from build123d import *

# Parameters (mm, degrees)
SKETCH1_W                 = 50.8
SKETCH1_H                 = 76.2
BOSS_EXTRUDE1_DEPTH       = 2.9972
SKETCH2_W                 = 2.9972
SKETCH2_H                 = 12.7
BOSS_EXTRUDE2_DEPTH       = 2.9972
F_8_CLEARANCE_HOLE1_D     = 4.3053
F_8_CLEARANCE_HOLE1_DEPTH = 6.351016
SKETCH6_R                 = 4.7625
CUT_EXTRUDE1_DEPTH        = 48.612962265


with BuildPart() as part:
    # Sketch1 → Boss-Extrude1 (new body)
    with BuildSketch(Plane(origin=(0, 0, 0), x_dir=(1, 0, 0), z_dir=(0, 1, 0))):
        Rectangle(SKETCH1_W, SKETCH1_H)
    extrude(amount=BOSS_EXTRUDE1_DEPTH)

    # Sketch2 → Boss-Extrude2 (add)
    with BuildSketch(Plane(origin=(0, 2.9972, 0), x_dir=(1, 0, 0), z_dir=(0, 1, 0))):
        with Locations((26.8986, 31.75)):
            Rectangle(SKETCH2_W, SKETCH2_H)
        with Locations((26.8986, -31.75)):
            Rectangle(SKETCH2_W, SKETCH2_H)
        with Locations((-26.8986, -31.75)):
            Rectangle(SKETCH2_W, SKETCH2_H)
        with Locations((-26.8986, 31.75)):
            Rectangle(SKETCH2_W, SKETCH2_H)
    extrude(amount=-BOSS_EXTRUDE2_DEPTH)

    # #8 Clearance Hole1
    with Locations(Plane(origin=(0, 2.9972, 0), x_dir=(1, 0, 0), z_dir=(0, 1, 0))):
        with Locations((12.7, -25.4), (0, -25.4), (-12.7, -25.4), (-12.7, -12.7), (0, -12.7), (12.7, -12.7), (-12.7, 0), (0, 0), (12.7, 0), (12.7, 12.7), (0, 12.7), (-12.7, 12.7), (-12.7, 25.4), (0, 25.4), (12.7, 25.4)):
            Hole(F_8_CLEARANCE_HOLE1_D / 2, depth=F_8_CLEARANCE_HOLE1_DEPTH)

    # Sketch6 → Cut-Extrude1 (cut, through all)
    with BuildSketch(Plane(origin=(0, 2.9972, 0), x_dir=(1, 0, 0), z_dir=(0, 1, 0))):
        with Locations(Location((0, 0, 0), (0, 0, 270))):
            Circle(SKETCH6_R)
    extrude(amount=-CUT_EXTRUDE1_DEPTH, mode=Mode.SUBTRACT)


solid = part.part
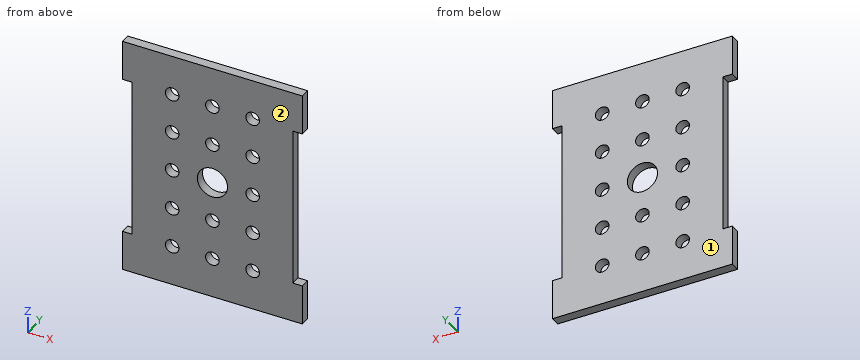
Build history of the part. All positions in model axes, mm. Face numbers are marked on the shaded views. Coordinates: 2 decimals unless noted, no trailing zeros. Write each loop counter-clockwise with the first axis right and the second up, starting at its lowest first coordinate (ties: lowest second). Pieces come first, ordered by that corner, then holes. Notation, with made-up numbers: (7.5, 43) -> (18.5, 43) arc R32 cw to (18.5, 80) -> close; hole circle Ø11 at (-27.75, 24.5). An arc over 180 degrees is marked (long way). Use CSV: the item, a comma, the result in double quotes. Start each with the question number.
Q1. Cut at A-A, the plane x = 0. List the corners of the cut face in (y, z).
Q2. Cut at C-C, the plane y = 2.45. State how many separate pieces and enclosed holes the cut face has, then the cut area to 3 significant figures.
Q3. Cut at B-B, the plane z = 0. List the corners of the cut face in (x, y), then the cut area to 3 significant figures.
Q4. Cut at D-D, the plane x = 12.7. List the corners of the cut face in (y, z), then the cut area to 3 significant figures.
Q5. Drill centre lines: probe 1 along Z at (x, y) = (12.7, 2.25); probe 2 along X at (y, z) = (0.8, -12.7); probe 3 along Z at (x, y) = (-11, 2.3). Where is each one in solid material? Low to high.
Q6. Flat gauge pins, fed straight in: pin 1 Ø3.5 at (x, z) = (0, -12.7) entering from +Y; pin 2 Ø7 at (x, z) = (12.7, 0) entering from -Y; pin 3 Ø0.9 at (y, z) = (1, 12) entering from -X. Where does each tip first touch, or does it go through?
Q7. Pull direction Y, two halves, no side cores. Call the marked faces 1 and 2: released by +Y, released by -Y, zero draft, split by the parting line, or undercut.
Checked values:
1,outline,"(0, -38.1) -> (3, -38.1) -> (3, -27.55) -> (0, -27.55) -> close; (0, -23.25) -> (3, -23.25) -> (3, -14.85) -> (0, -14.85) -> close; (0, -10.55) -> (3, -10.55) -> (3, -4.76) -> (0, -4.76) -> close; (0, 4.76) -> (3, 4.76) -> (3, 10.55) -> (0, 10.55) -> close; (0, 14.85) -> (3, 14.85) -> (3, 23.25) -> (0, 23.25) -> close; (0, 27.55) -> (3, 27.55) -> (3, 38.1) -> (0, 38.1) -> close"
2,separate pieces,"1"
2,enclosed holes,"15"
2,area,"3,750 mm²"
3,outline,"(-25.4, 0) -> (-14.85, 0) -> (-14.85, 3) -> (-25.4, 3) -> close; (-10.55, 0) -> (-4.76, 0) -> (-4.76, 3) -> (-10.55, 3) -> close; (4.76, 0) -> (10.55, 0) -> (10.55, 3) -> (4.76, 3) -> close; (14.85, 0) -> (25.4, 0) -> (25.4, 3) -> (14.85, 3) -> close"
3,area,"97.9 mm²"
4,outline,"(0, -38.1) -> (3, -38.1) -> (3, -27.55) -> (0, -27.55) -> close; (0, -23.25) -> (3, -23.25) -> (3, -14.85) -> (0, -14.85) -> close; (0, -10.55) -> (3, -10.55) -> (3, -2.15) -> (0, -2.15) -> close; (0, 2.15) -> (3, 2.15) -> (3, 10.55) -> (0, 10.55) -> close; (0, 14.85) -> (3, 14.85) -> (3, 23.25) -> (0, 23.25) -> close; (0, 27.55) -> (3, 27.55) -> (3, 38.1) -> (0, 38.1) -> close"
4,area,"164 mm²"
5,probe 1,"z = -38.1 to -27.55, -23.25 to -14.85, -10.55 to -2.15, 2.15 to 10.55, 14.85 to 23.25, 27.55 to 38.1"
5,probe 2,"x = -25.4 to -14.85, -10.55 to -2.15, 2.15 to 10.55, 14.85 to 25.4"
5,probe 3,"z = -38.1 to -26.72, -24.08 to -14.02, -11.38 to -1.32, 1.32 to 11.38, 14.02 to 24.08, 26.72 to 38.1"
6,pin 1,"passes through"
6,pin 2,"stops at y = 0"
6,pin 3,"stops at x = -25.4"
7,face 1,"released by +Y"
7,face 2,"released by -Y"
